from build123d import *

# Parameters (mm, degrees)
SKETCH_W        = 42.3
SKETCH_H        = 40.3
SKETCH_R        = 12
SKETCH_R_2      = 1.7
PAD_DEPTH       = 3
CHAMFER_SIZE    = 5
SKETCH001_W     = 5
SKETCH001_H     = 20
PAD001_DEPTH    = 5
SKETCH002_R     = 1.7
POCKET_DEPTH    = 42.301
POCKET001_DEPTH = 1.5
SKETCH004_R     = 1.7
PAD002_DEPTH    = 2
SKETCH005_W     = 47.453737
SKETCH005_H     = 16.482529
POCKET002_DEPTH = 50


with BuildPart() as part:
    # Sketch → Pad (new body)
    with BuildSketch(Plane.XY):
        Rectangle(SKETCH_W, SKETCH_H)
        Circle(SKETCH_R, mode=Mode.SUBTRACT)
        with Locations((-15.5, 15.5)):
            Circle(SKETCH_R_2, mode=Mode.SUBTRACT)
        with Locations((-15.5, -15.5)):
            Circle(SKETCH_R_2, mode=Mode.SUBTRACT)
        with Locations((15.5, -15.5)):
            Circle(SKETCH_R_2, mode=Mode.SUBTRACT)
        with Locations((15.5, 15.5)):
            Circle(SKETCH_R_2, mode=Mode.SUBTRACT)
    extrude(amount=PAD_DEPTH)

    # Chamfer
    chamfer_edges = [part.edges().sort_by_distance(p)[0] for p in [
        (21.15, -20.15, 1.5),
        (-21.15, -20.15, 1.5),
        (21.15, 20.15, 1.5),
        (-21.15, 20.15, 1.5),
    ]]
    chamfer(chamfer_edges, length=CHAMFER_SIZE)

    # Sketch001 (on Face5 of Chamfer) → Pad001 (join)
    with BuildSketch(Plane.XY.offset(3)):
        with Locations((-18.65, 0)):
            Rectangle(SKETCH001_W, SKETCH001_H)
    extrude(amount=PAD001_DEPTH)

    # Sketch002 (on Face19 of Pad001) → Pocket (cut, through all)
    with BuildSketch(Plane(origin=(-21.15, 0, 0), x_dir=(0, -1, 0), z_dir=(-1, 0, 0))):
        with Locations((-4.5, 5)):
            Circle(SKETCH002_R)
        with Locations((4.5, 5)):
            Circle(SKETCH002_R)
    extrude(amount=-POCKET_DEPTH, mode=Mode.SUBTRACT)

    # Sketch003 (on DatumPlane) → Pocket001 (cut, symmetric)
    with BuildSketch(Plane(origin=(-18.65, 0, 0), x_dir=(0, -1, 0), z_dir=(-1, 0, 0))):
        Polygon((4.5, 1.65), (7.401185, 3.325), (7.401185, 13.325), (1.598815, 13.325), (1.598815, 3.325), align=None)
        Polygon((-4.5, 1.65), (-1.598815, 3.325), (-1.598815, 13.325), (-7.401185, 13.325), (-7.401185, 3.325), align=None)
    extrude(amount=POCKET001_DEPTH, both=True, mode=Mode.SUBTRACT)

    # Sketch004 (on Face6 of Pocket001) → Pad002 (join)
    with BuildSketch(Plane(origin=(-21.15, 0, 0), x_dir=(0, -1, 0), z_dir=(-1, 0, 0))):
        Polygon((15, -33), (-15, -33), (-15, 3), (-10, 3), (-10, 8), (10, 8), (10, 3), (15, 3), align=None)
        with Locations((-4.5, 5)):
            Circle(SKETCH004_R, mode=Mode.SUBTRACT)
        with Locations((4.5, 5)):
            Circle(SKETCH004_R, mode=Mode.SUBTRACT)
    extrude(amount=PAD002_DEPTH)

    # Sketch005 (on Face1 of Pad002) → Pocket002 (cut)
    with BuildSketch(Plane(origin=(0, 20.15, 0), x_dir=(-1, 0, 0), z_dir=(0, 1, 0))):
        with Locations((-2.626869, 2.50214)):
            Rectangle(SKETCH005_W, SKETCH005_H)
    extrude(amount=-POCKET002_DEPTH, mode=Mode.SUBTRACT)


solid = part.part
Source: CAD feature listing. Evaluate the final solid. Frame: model axes, mm. A direction names the side the tool comes from. Round coordinates to 2 decimals unless told otherwise and drop trailing zeros. Loops run counter-clockwise (first coordinate to the right, second up) from the corner with the lowest first, then second, coordinate; pieces in that order, holes last.
Q1. First-contact query: P1, Ø12, axis at y = -7.5, z = -26.5, coming from the +X side; P2, Ø0.6, axis at x = -22.5, z = 6.5, coming from the -Y side; P3, Ø0.6, axis at x = -22, z = -10, coming from the -Y side. Flat tips, straight axial feed; report the tip coordinate or a pass-through.
Q2. Access query for faces 1 (the face through (-21.15, 0, -16)), 2 (the face through (-23.15, 0, -12)), 3 (the face through (-22, 13, 3)), 4 (the face through (-22, -13, 3)), 5 (the face through (-21.1, 0, 3)). Directions: +Z, -Z, +X, -X, +Y, -Y. A direction counts if a zero-diameter tool reaches every point of the face in a straight line with its end or side. Return the directions, or none.
Q3. Section B-B, the plane y = -4.5. Return loops of the section in (x, z), plus the area to 3 significant figures.
Q4. Ray query, line 1 (Z direction, x = -21.95, y = 4.5); line 2 (Y direction, x = -22.8, z = -12.5); line 3 (X direction, y = -5.5, z = -8). Return the intervals inside material, ascending.
Q5. Section C-C, the plane z = 5. Return loops of the section in (x, y), plus the area to 3 significant figures.
Q6. Section A-A, the plane x = -22.55. Return loops of the section in (y, z), plus the area to 3 significant figures.
Q7. Section D-D, the plane z = -18.5. Return loops of the section in (x, y), plus the area to 3 significant figures.
Solutions:
1. P1: stops at x = -21.15
1. P2: stops at y = -10
1. P3: stops at y = -15
2. face 1: -Z, +X, +Y, -Y
2. face 2: +Z, -Z, -X, +Y, -Y
2. face 3: +Z, +X, -X, +Y
2. face 4: +Z, +X, -X, -Y
2. face 5: +Z, -Z, +X, +Y, -Y
3. outline: (-23.15, -33) - (-21.15, -33) - (-21.15, 0) - (-21.1, 0) - (-21.1, 3.3) - (-23.15, 3.3) - close; (-23.15, 6.7) - (-21.1, 6.7) - (-21.1, 8) - (-23.15, 8) - close
3. area: 75.4 mm2
4. line 1: z = -33 to 3.3, 6.7 to 8
4. line 2: y = -15 to 15
4. line 3: x = -23.15 to -21.15
5. outline: (-23.15, -10) - (-21.1, -10) - (-21.1, -6.2) - (-23.15, -6.2) - close; (-23.15, -2.8) - (-21.1, -2.8) - (-21.1, 2.8) - (-23.15, 2.8) - close; (-23.15, 6.2) - (-21.1, 6.2) - (-21.1, 10) - (-23.15, 10) - close
5. area: 27.1 mm2
6. outline: (-15, -33) - (15, -33) - (15, 3) - (10, 3) - (10, 8) - (-10, 8) - (-10, 3) - (-15, 3) - close; hole circle Ø3.4 at (-4.5, 5); hole circle Ø3.4 at (4.5, 5)
6. area: 1,160 mm2
7. outline: (-23.15, -15) - (-21.15, -15) - (-21.15, 15) - (-23.15, 15) - close
7. area: 60.0 mm2
